from build123d import *

# Parameters (mm, degrees)
F0_R     = 10.35
F1_DEPTH = 10
F2_R     = 1
F3_R     = 3.65
F4_DEPTH = 25
F5_R     = 10.3
F6_DEPTH = 8.9
F8_DEPTH = 12.5


with BuildPart() as f1:
    # F0 (on Top) → F1 (new body)
    with BuildSketch(Plane.XY):
        Circle(F0_R)
    extrude(amount=F1_DEPTH)

    # F2
    f2_edges = [f1.edges().sort_by_distance(p)[0] for p in [
        (-10.35, 0, 10),
    ]]
    fillet(f2_edges, radius=F2_R)

    # F3 (on face) → F4 (cut)
    with BuildSketch(Plane.XY.offset(10)):
        Circle(F3_R)
    extrude(amount=-F4_DEPTH, mode=Mode.SUBTRACT)

    # F5 (on face) → F6 (cut)
    with BuildSketch(Plane(origin=(0, 0, 0), x_dir=(1, 0, 0), z_dir=(0, 0, -1))):
        Circle(F5_R)
    extrude(amount=-F6_DEPTH, mode=Mode.SUBTRACT)

    # F7 (on Front) → F8 (cut, symmetric)
    with BuildSketch(Plane.XZ):
        with BuildLine():
            ThreePointArc((0, 3), (1.06066, 3.43934), (1.5, 4.5))
            ThreePointArc((1.5, 4.5), (-1.06066, 5.56066), (0, 3))
        make_face()
    extrude(amount=F8_DEPTH, both=True, mode=Mode.SUBTRACT)


solid = f1.part
Read the model definition and answer for the solid it produces. Units are mm, in the model's axes. Coordinates: 2 decimals unless noted, no trailing zeros. Order: outer loops, then holes, each group sorted by start corner. A loop starts at its lowest first (then second) coordinate and runs counter-clockwise, first axis right, second up. Notation, with made-up numbers: M 31.5,-22 L 80.5,-22 A31 cw 80.5,11 Z; hole C 59,-20 d8. An arc over 180 degrees is marked long. Put each result on its own line as item: value. Start each with the question number.
Item 1: Section B-B, the plane z = 2 is taken. Determine the outline of the cut face in (x, y).
Item 2: Consider probe 1 along Z at (x, y) = (-8.5, 0.75); probe 2 along X at (y, z) = (3.25, 9); probe 3 along X at (y, z) = (1, 9.5). Determine where each line is inside the solid, lowest interval first. Write a range as [from, to].
Item 3: The mould has two halves that part along Y. Classify faces 1 (the face through (0, -4, 10)), 2 (the face through (0, 4, 8.9)): +Y half, -Y half, draft (parallel to the pull), parting line (faces both ways), or undercut.
Item 4: Given pin 1 Ø2 at (x, z) = (-4.5, 5.5) entering from -Y; pin 2 Ø4.5 at (x, y) = (0, 0) entering from -Z; pin 3 Ø5 at (y, z) = (-7, 2) entering from +X; pin 4 Ø6 at (x, z) = (-5, 7) entering from -Y, each flat-ended and moving along its own axis, determine where each tip first touches the part or whether it passes through.
Item 5: Section A-A, the plane y = 0 is taken. Determine the outline of the cut face in (x, z), plus the area to 3 significant figures.
Computed:
1. outline: C 0,0 d20.7; hole C 0,0 d20.6
2. probe 1: z = [8.9, 10]
2. probe 2: x = [-9.83, -1.66], [1.66, 9.83]
2. probe 3: x = [-10.17, -3.51], [3.51, 10.17]
3. face 1: draft
3. face 2: undercut
4. pin 1: stops at y = -9.74
4. pin 2: passes through
4. pin 3: stops at x = 9.32
4. pin 4: stops at y = -10.15
5. outline: M -10.35,0 L -10.3,0 L -10.3,8.9 L -3.65,8.9 L -3.65,10 L -9.35,10 A1 ccw -10.35,9 Z; M 3.65,8.9 L 10.3,8.9 L 10.3,0 L 10.35,0 L 10.35,9 A1 ccw 9.35,10 L 3.65,10 Z
5. area: 15.2 mm2
